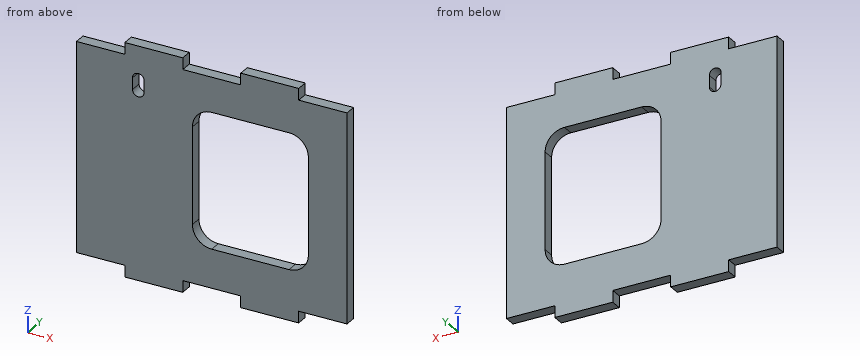
```python
from build123d import *

# Parameters (mm, degrees)
BOSS_EXTRUDE1_DEPTH = 3
CUT_EXTRUDE1_DEPTH  = 47.19523785
CUT_EXTRUDE3_DEPTH  = 47.19523785


with BuildPart() as part:
    # Sketch1 → Boss-Extrude1 (new body)
    with BuildSketch(Plane(origin=(0, 0, 0), x_dir=(1, 0, 0), z_dir=(0, 1, 0))):
        Polygon((-35, 27), (-22.5, 27), (-22.5, 30), (-7.5, 30), (-7.5, 27), (7.5, 27), (7.5, 30), (22.5, 30), (22.5, 27), (35, 27), (35, -27), (22.5, -27), (22.5, -30), (7.5, -30), (7.5, -27), (-7.5, -27), (-7.5, -30), (-22.5, -30), (-22.5, -27), (-35, -27), align=None)
    extrude(amount=BOSS_EXTRUDE1_DEPTH)

    # Sketch2 → Cut-Extrude1 (cut, through all)
    with BuildSketch(Plane(origin=(0, 3, 0), x_dir=(1, 0, 0), z_dir=(0, 1, 0))):
        with BuildLine():
            Line((0, 17), (20, 17))
            ThreePointArc((20, 17), (23.535533906, 15.535533906), (25, 12))
            Line((25, 12), (25, -13))
            ThreePointArc((25, -13), (23.535533906, -16.535533906), (20, -18))
            Line((20, -18), (0, -18))
            ThreePointArc((0, -18), (-3.535533906, -16.535533906), (-5, -13))
            Line((-5, -13), (-5, 12))
            ThreePointArc((-5, 12), (-3.535533906, 15.535533906), (0, 17))
        make_face()
    extrude(amount=-CUT_EXTRUDE1_DEPTH, mode=Mode.SUBTRACT)

    # Sketch4 → Cut-Extrude3 (cut, through all)
    with BuildSketch(Plane(origin=(0, 3, 0), x_dir=(1, 0, 0), z_dir=(0, 1, 0))):
        with BuildLine():
            Line((-17.5, -18.5), (-17.5, -21.5))
            ThreePointArc((-17.5, -21.5), (-19, -23), (-20.5, -21.5))
            Line((-20.5, -21.5), (-20.5, -18.5))
            ThreePointArc((-20.5, -18.5), (-19, -17), (-17.5, -18.5))
        make_face()
    extrude(amount=-CUT_EXTRUDE3_DEPTH, mode=Mode.SUBTRACT)


solid = part.part
```
Work out the finished part from the listing and answer in its coordinate system (mm). Give positions to 0.01 mm unless a question says otherwise; leave off trailing zeros. Order: outer loops, then holes, each group sorted by start corner. A loop starts at its lowest first (then second) coordinate and runs counter-clockwise, first axis right, second up. Notation, with made-up numbers: (89.5, 16.5) - (144.5, 16.5) arc R14 cw to (144.5, 41.5) - close; hole circle Ø1 at (59, 85). An arc over 180 degrees is marked (long way). One line per item, written item: value. Start each with the question number.
1. Consider line 1 (X direction, y = 0.9, z = 20); line 2 (Z direction, x = 0.5, y = 1.5); line 3 (X direction, y = 2, z = 8). Determine where each line is inside the solid, lowest interval first.
2. Section A-A, the plane x = 18.5 is taken. Write down the section's boundary in (y, z), then the cut area to 3 significant figures.
3. Section C-C, the plane y = 0.7 is taken. Count the separate pieces of the cut face and the enclosed holes in it, then the cut area to 3 significant figures.
4. Each of these flat-tipped pins is pushed along its axis until it touches: pin 1 Ø10 at (x, z) = (15.5, -8.5) entering from +Y; pin 2 Ø0.9 at (y, z) = (1.5, 28.5) entering from +X; pin 3 Ø1.5 at (y, z) = (1.5, -28) entering from -X; pin 4 Ø1.5 at (x, y) = (1, 1.5) entering from +Z. Where does it stop, or does it pass through?
5. Section B-B, the plane z = -15 is taken. Write down the section's boundary in (x, y), then the cut area to 3 significant figures.
6. Section D-D, the plane x = -26 is taken. Write down the section's boundary in (y, z).
Filled sheet:
1. line 1: -35 to -20.5, -17.5 to 35
1. line 2: -27 to -17, 18 to 27
1. line 3: -35 to -5, 25 to 35
2. outline: (0, -30) - (3, -30) - (3, -17) - (0, -17) - close; (0, 18) - (3, 18) - (3, 30) - (0, 30) - close
2. area: 75.0 mm²
3. separate pieces: 1
3. enclosed holes: 2
3. area: 2,920 mm²
4. pin 1: through
4. pin 2: x = 22.5
4. pin 3: x = -22.5
4. pin 4: z = 27
5. outline: (-35, 0) - (-4, 0) - (-4, 3) - (-35, 3) - close; (24, 0) - (35, 0) - (35, 3) - (24, 3) - close
5. area: 126 mm²
6. outline: (0, -27) - (3, -27) - (3, 27) - (0, 27) - close
